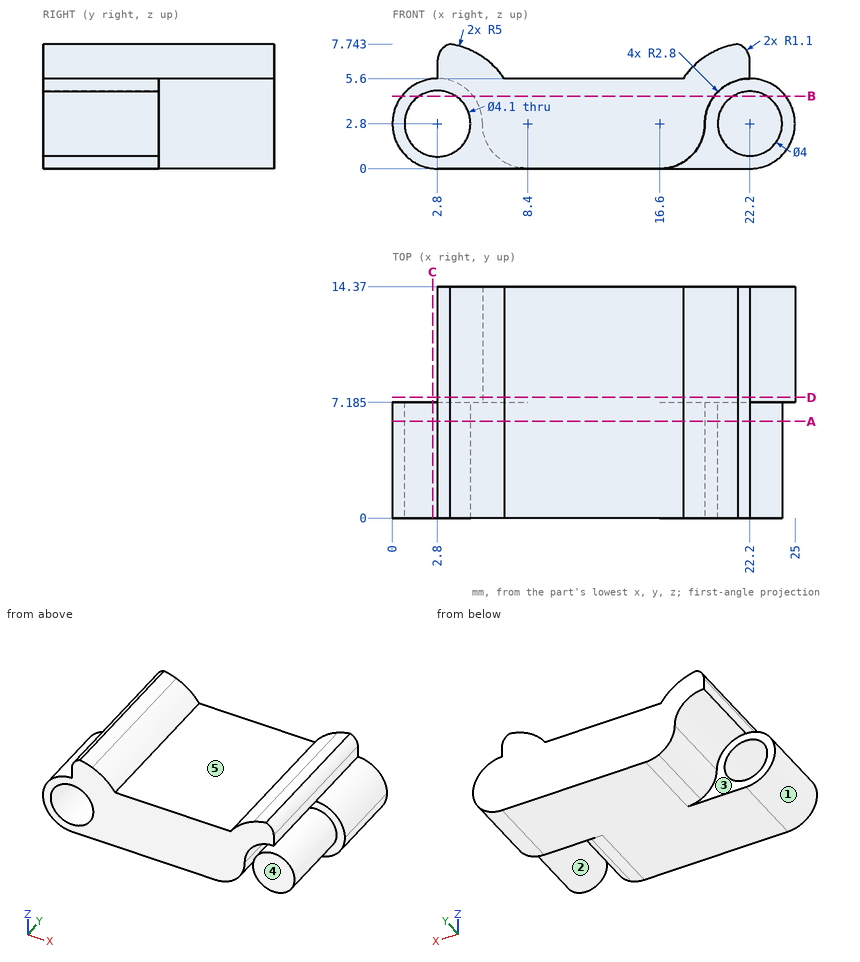
Print and shaded views of the part. All mm, measured from the part's lowest x, y and z. A direction names the side the tool comes from. Give positions to 0.01 mm unless a question says otherwise; leave off trailing zeros. Loops run counter-clockwise (first coordinate to the right, second up) from the corner with the lowest first, then second, coordinate; pieces in that order, holes last. Notation, with made-up numbers: (-11, 53) -> (29, 53) arc R15 cw to (29, 59) -> close; hole circle Ø1 at (-17, 22.5). An arc over 180 degrees is marked (long way). One line per question, with ' | ' between items. Start each with the question number.
1) 3-axis set-ups, long thin cutter, end or side, ignore diameter. For the marked faces 4 and 5: which of +Z, -Z, +X, -X, +Y, -Y reach the whole face in a straight line?
2) Cut at C-C (x = 2.5). Give the cut face in (y, z) (1 decimal).
3) Pin check, flat tips, straight feed: pin 1 (3.5 mm diameter, centred on x = 2.8, z = 2.8, fed in from +Y); pin 2 (0.9 mm diameter, centred on y = 10.5, z = 6.5, fed in from +X); pin 3 (1 mm diameter, centred on y = 12, z = 1.5, fed in from -X); pin 4 (1.2 mm diameter, centred on y = 7, z = 6.5, fed in from -X). Stop position of each tip, or through.
4) Probe L1, parallel to X at y = 7, z = 2.75; L2, parallel to X at y = 1, z = 4; L3, parallel to Z at x = 14, y = 4. List the from-to ranges inside material, lowest first.
5) Cut at A-A (y = 6). Give the cut face in (x, z).
6) Cut at B-B (z = 4.5). Give the cut face in (x, y) (1 decimal).
7) Cut at D-D (y = 7.5). Give the cut face in (x, z), plus the area to 3 significant figures.
8) Two-plate mould, pull along X, no slides. Class the marked faces 1, 2 and 3: released by +X, released by -X, zero draft, split by the parting line, or undercut.
Return value:
1) face 4: +Z, -Z, +X, -X, -Y | face 5: +Z, +Y, -Y
2) outline: (0, 0) -> (7.2, 0) -> (7.2, 0.8) -> (0, 0.8) -> close; (0, 4.8) -> (7.2, 4.8) -> (7.2, 5.6) -> (0, 5.6) -> close
3) pin 1: through | pin 2: x = 22.2 | pin 3: x = 5.72 | pin 4: x = 2.8
4) L1: 0 to 0.75, 4.85 to 19.4, 20.2 to 24.2 | L2: 0.27 to 1.14, 4.46 to 19.67, 20.6 to 23.8 | L3: 0 to 5.6
5) outline: (2.8, 0) -> (16.6, 0) arc R2.8 ccw to (19.4, 2.8) arc R2.8 cw to (22.2, 5.6) -> (22.2, 6.7) arc R1.1 ccw to (21.45, 7.74) arc R5 ccw to (18.06, 5.6) -> (6.94, 5.6) arc R5 ccw to (3.55, 7.74) arc R1.1 ccw to (2.8, 6.7) -> (2.8, 5.6) arc R2.8 ccw to start; circle Ø4 at (22.2, 2.8); hole circle Ø4.1 at (2.8, 2.8)
6) outline: (0.6, 0) -> (1.7, 0) -> (1.7, 7.2) -> (0.6, 7.2) -> close; (3.9, 0) -> (20, 0) -> (20, 7.2) -> (21.1, 7.2) -> (21.1, 0) -> (23.3, 0) -> (23.3, 7.2) -> (24.4, 7.2) -> (24.4, 14.4) -> (5, 14.4) -> (5, 7.2) -> (3.9, 7.2) -> close
7) outline: (2.8, 5.6) arc R2.8 cw to (5.6, 2.8) arc R2.8 ccw to (8.4, 0) -> (22.2, 0) arc R2.8 ccw to (22.2, 5.6) -> (22.2, 6.7) arc R1.1 ccw to (21.45, 7.74) arc R5 ccw to (18.06, 5.6) -> (6.94, 5.6) arc R5 ccw to (3.55, 7.74) arc R1.1 ccw to (2.8, 6.7) -> close | area: 118 mm^2
8) face 1: released by -X | face 2: undercut | face 3: zero draft
